```python
from build123d import *

# Parameters (mm, degrees)
F1_DEPTH  = 12
F2_R      = 29.5
F3_DEPTH  = 12
F3_FACE_R = 29.5
F5_R      = 19.5
F7_DEPTH  = 4.5
F8_R      = 18.5
F9_DEPTH  = 4.5
F10_R     = 15
F11_DEPTH = 10
F12_R     = 10
F13_DEPTH = 48.001


with BuildPart() as f1:
    # F0 (on Front) → F1 (new body)
    with BuildSketch(Plane.XZ):
        with BuildLine():
            Line((-32, 0), (32, 0))
            ThreePointArc((32, 0), (0, 32), (-32, 0))
        make_face()
        with BuildLine():
            Line((32, -39), (32, 0))
            Line((32, 0), (-32, 0))
            Line((-32, 0), (-32, -39))
            Line((-32, -39), (-31.5, -39))
            ThreePointArc((-31.5, -39), (-29.3786796564, -39.8786796564), (-28.5, -42))
            Line((-28.5, -42), (-28.5, -52))
            Line((-28.5, -52), (28.5, -52))
            Line((28.5, -52), (28.5, -42))
            ThreePointArc((28.5, -42), (29.3786796564, -39.8786796564), (31.5, -39))
            Line((31.5, -39), (32, -39))
        make_face()
    extrude(amount=F1_DEPTH)

    # F2 (on face) → F3 (join)
    with BuildSketch(Plane.XZ.offset(12)):
        Circle(F2_R)
    extrude(amount=F3_DEPTH)

    # F3_face (on face) → F6 section 0
    with BuildSketch(Plane.XZ.offset(24)):
        Circle(F3_FACE_R)
    # F5 (on offset) → F6 section 1
    with BuildSketch(Plane.XZ.offset(29)):
        Circle(F5_R)
    loft()

    # F7 (add): a face of the model
    f7_faces = [f1.faces().sort_by_distance(p)[0] for p in [
        (0, -29, 0),
    ]]
    extrude(f7_faces, amount=F7_DEPTH)

    # F8 (on face) → F9 (join)
    with BuildSketch(Plane.XZ.offset(33.5)):
        Circle(F8_R)
    extrude(amount=F9_DEPTH)

    # F10 (on face) → F11 (join)
    with BuildSketch(Plane.XZ.offset(38)):
        Circle(F10_R)
    extrude(amount=F11_DEPTH)

    # F12 (on face) → F13 (cut, through all)
    with BuildSketch(Plane.XZ.offset(48)):
        Circle(F12_R)
    extrude(amount=-F13_DEPTH, mode=Mode.SUBTRACT)


solid = f1.part
```
Source: CAD feature listing. Evaluate the final solid. Frame: model axes, mm. A direction names the side the tool comes from. Round coordinates to 2 decimals unless told otherwise and drop trailing zeros. Loops run counter-clockwise (first coordinate to the right, second up) from the corner with the lowest first, then second, coordinate; pieces in that order, holes last.
(1) Section query C-C (z = -32). Output: boundary loops of the cut face in (x, y).
From the geometry:
outline: (-32, -12) - (32, -12) - (32, 0) - (-32, 0) - close
(2) Section query D-D (y = -20.5). Output: boundary loops of the cut face in (x, z), and give its area (3 significant figures).
From the geometry:
outline: circle Ø59 at (0, 0); hole circle Ø20 at (0, 0)
area: 2,420 mm2
(3) Section query B-B (y = -37). Output: boundary loops of the cut face in (x, z).
From the geometry:
outline: circle Ø37 at (0, 0); hole circle Ø20 at (0, 0)
(4) Material intervals for probe 1 along Z at (x, y) = (0, -31); probe 2 along Z at (x, y) = (0, -16.5); probe 3 along X at (y, z) = (-42, -8.5), sorted ascending.
From the geometry:
probe 1: z = -19.5 to -10, 10 to 19.5
probe 2: z = -29.5 to -10, 10 to 29.5
probe 3: x = -12.36 to -5.27, 5.27 to 12.36
(5) Contact query for flat-ended pins moving along their axis: pin 1 Ø2 at (y, z) = (-27, -10.5) entering from +X; pin 2 Ø1 at (y, z) = (-21, 19) entering from -X; pin 3 Ø11 at (y, z) = (-7.5, -45) entering from -X. Output: stop coordinate, or through.
From the geometry:
pin 1: stops at x = 23.28
pin 2: stops at x = -22.98
pin 3: stops at x = -29.84
(6) Access query for faces 1 (the flat face through (-28.5, -6, -47)), 2 (the flat face through (28.5, -6, -47)), 3 (the cylindrical face through (-2.539, -31.218, 19.334)), 4 (the flat face through (0, 0, -19)), 5 (the flat face through (3, -48, -10)). Directions: +Z, -Z, +X, -X, +Y, -Y. A direction counts if a zero-diameter tool reaches every point of the face in a straight line with its end or side. Return the directions, or none.
From the geometry:
face 1: -Z, -X, +Y, -Y
face 2: -Z, +X, +Y, -Y
face 3: -Y
face 4: +Z, -Z, +X, -X, +Y
face 5: +Z, -Z, +X, -X, -Y
(7) Pull-direction query (X, two-part tool) for faces 6 (the conical face through (10.74, -28.76, 16.85)), 7 (the cylindrical face through (-2.17, -24.34, -9.76)), 8 (the flat face through (-32, -6, -19)); classes: +X half, -X half, draft (parallel to the pull), parting line (faces both ways), or undercut.
From the geometry:
face 6: parting line
face 7: undercut
face 8: -X half
(8) Section query A-A (x = 0). Output: boundary loops of the cut face in (y, z), and give its area (3 significant figures).
From the geometry:
outline: (-48, -15) - (-38, -15) - (-38, -18.5) - (-33.5, -18.5) - (-33.5, -19.5) - (-29, -19.5) - (-24, -29.5) - (-12, -29.5) - (-12, -52) - (0, -52) - (0, -10) - (-48, -10) - close; (-48, 10) - (0, 10) - (0, 32) - (-12, 32) - (-12, 29.5) - (-24, 29.5) - (-29, 19.5) - (-33.5, 19.5) - (-33.5, 18.5) - (-38, 18.5) - (-38, 15) - (-48, 15) - close
area: 1,640 mm2
